Build history of the part. All positions in model axes, mm. A direction names the side the tool comes from. Coordinates: 2 decimals unless noted, no trailing zeros. Write each loop counter-clockwise with the first axis right and the second up, starting at its lowest first coordinate (ties: lowest second). Pieces come first, ordered by that corner, then holes.
```python
from build123d import *

# Parameters (mm, degrees)
F0_W     = 57.99
F0_H     = 6.35
F0_H_2   = 44.45
F1_DEPTH = 6.35
F2_DEPTH = 44.45
F3_R     = 2
F4_DEPTH = 50.801


# Not quite as in the source:
# - a length typed as a fraction of an inch, garbled in the dataset ("3 / 203.2 mm" for 3/8 in), is restored
# - a feature names something its author has since deleted; it is built from what else it names


with BuildPart() as f1:
    # F0 (on Top) → F1 (new body)
    with BuildSketch(Plane.XY):
        with Locations((-9.895, 22.275)):
            Rectangle(F0_W, F0_H)
        with Locations((-9.895, -3.125)):
            Rectangle(F0_W, F0_H_2)
        with BuildLine():
            ThreePointArc((-17.1, -15.5), (-15.5, -13.9), (-13.9, -15.5))
            Line((-13.9, -15.5), (-13.9, -21.75))
            ThreePointArc((-13.9, -21.75), (-15.5, -23.35), (-17.1, -21.75))
            Line((-17.1, -21.75), (-17.1, -15.5))
        make_face(mode=Mode.SUBTRACT)
        with BuildLine():
            ThreePointArc((13.9, -15.5), (15.5, -13.9), (17.1, -15.5))
            Line((17.1, -15.5), (17.1, -21.75))
            ThreePointArc((17.1, -21.75), (15.5, -23.35), (13.9, -21.75))
            Line((13.9, -21.75), (13.9, -15.5))
        make_face(mode=Mode.SUBTRACT)
        with BuildLine():
            ThreePointArc((-11.1, 0), (0, 11.1), (11.1, 0))
            Line((11.1, 0), (11.1, -6.25))
            ThreePointArc((11.1, -6.25), (0, -17.35), (-11.1, -6.25))
            Line((-11.1, -6.25), (-11.1, 0))
        make_face(mode=Mode.SUBTRACT)
        with BuildLine():
            ThreePointArc((-17.1, 15.5), (-15.5, 17.1), (-13.9, 15.5))
            Line((-13.9, 15.5), (-13.9, 9.25))
            ThreePointArc((-13.9, 9.25), (-15.5, 7.65), (-17.1, 9.25))
            Line((-17.1, 9.25), (-17.1, 15.5))
        make_face(mode=Mode.SUBTRACT)
        with BuildLine():
            ThreePointArc((13.9, 15.5), (15.5, 17.1), (17.1, 15.5))
            Line((17.1, 15.5), (17.1, 9.25))
            ThreePointArc((17.1, 9.25), (15.5, 7.65), (13.9, 9.25))
            Line((13.9, 9.25), (13.9, 15.5))
        make_face(mode=Mode.SUBTRACT)
    extrude(amount=F1_DEPTH)

    # F0 (on Top) → F2 (join)
    with BuildSketch(Plane.XY):
        with Locations((-9.895, 22.275)):
            Rectangle(F0_W, F0_H)
    extrude(amount=-F2_DEPTH)

    # F3 (on face) → F4 (cut, through all)
    with BuildSketch(Plane(origin=(0, 25.45, 0), x_dir=(-1, 0, 0), z_dir=(0, 1, 0))):
        with Locations((28.89, -6)):
            Circle(F3_R)
        with Locations((28.89, -38.45)):
            Circle(F3_R)
    extrude(amount=-F4_DEPTH, mode=Mode.SUBTRACT)


solid = f1.part
```
1. Saw through at C-C on y = -9. List the corners of the cut face in (x, z), plus the area to 3 significant figures.
Computed values:
outline: (-38.89, 0) - (-10.75, 0) - (-10.75, 6.35) - (-38.89, 6.35) - close; (10.75, 0) - (19.1, 0) - (19.1, 6.35) - (10.75, 6.35) - close
area: 232 mm2
2. Saw through at A-A on x = -15.5. List the corners of the cut face in (y, z), plus the area to 3 significant figures.
Computed values:
outline: (-25.35, 0) - (-23.35, 0) - (-23.35, 6.35) - (-25.35, 6.35) - close; (-13.9, 0) - (7.65, 0) - (7.65, 6.35) - (-13.9, 6.35) - close; (17.1, 0) - (19.1, 0) - (19.1, -44.45) - (25.45, -44.45) - (25.45, 6.35) - (17.1, 6.35) - close
area: 485 mm2
3. Probe line 1 along Z through (x, y) = (-28.89, 22.75); line 2 along Z through (x, y) = (-28, 20); line 3 along Z through (x, y) = (-24, 3.5). List the from-to ranges inside material, lowest first.
Computed values:
line 1: z = -44.45 to -40.45, -36.45 to -8, -4 to 6.35
line 2: z = -44.45 to -40.24, -36.66 to -7.79, -4.21 to 6.35
line 3: z = 0 to 6.35
4. Flat gauge pins, fed straight in: pin 1 (2 mm diameter, centred on x = -26, y = 8.5, fed in from -Z); pin 2 (6 mm diameter, centred on x = 8.5, z = -22.5, fed in from -Y). Where does each tip first touch, or does it go through?
Computed values:
pin 1: stops at z = 0
pin 2: stops at y = 19.1
5. Mould opens along Y. For faces 4 (the face through (-15.5, -13.9, 3.1)), 5 (the face through (-10, 25.45, -19)), 6 (the face through (-10, -25.35, 3)) say: +Y half, -Y half, draft (parallel to the pull), parting line (faces both ways), or undercut.
Computed values:
face 4: undercut
face 5: +Y half
face 6: -Y half
6. Saw through at D-D on z = -6. List the corners of the cut face in (x, y).
Computed values:
outline: (-38.89, 19.1) - (-30.89, 19.1) - (-30.89, 25.45) - (-38.89, 25.45) - close; (-26.89, 19.1) - (19.1, 19.1) - (19.1, 25.45) - (-26.89, 25.45) - close
7. 3-axis set-ups, long thin cutter, end or side, ignore diameter. For faces 1 (the face through (-38.89, 9, 2)), 2 (the face through (-15.5, 17.1, 3.1)), 3 (the face through (-10, 19.1, -22)): which of +Z, -Z, +X, -X, +Y, -Y reach the whole face in a straight line?
Computed values:
face 1: +Z, -Z, -X, +Y, -Y
face 2: +Z, -Z
face 3: -Z, +X, -X, -Y
8. Saw through at B-B on z = 2. List the corners of the cut face in (x, y), plus the area to 3 significant figures.
Computed values:
outline: (-38.89, -25.35) - (19.1, -25.35) - (19.1, 25.45) - (-38.89, 25.45) - close; hole (-17.1, -21.75) arc R1.6 ccw to (-13.9, -21.75) - (-13.9, -15.5) arc R1.6 ccw to (-17.1, -15.5) - close; hole (-17.1, 9.25) arc R1.6 ccw to (-13.9, 9.25) - (-13.9, 15.5) arc R1.6 ccw to (-17.1, 15.5) - close; hole (-11.1, -6.25) arc R11.1 ccw to (11.1, -6.25) - (11.1, 0) arc R11.1 ccw to (-11.1, 0) - close; hole (13.9, -21.75) arc R1.6 ccw to (17.1, -21.75) - (17.1, -15.5) arc R1.6 ccw to (13.9, -15.5) - close; hole (13.9, 9.25) arc R1.6 ccw to (17.1, 9.25) - (17.1, 15.5) arc R1.6 ccw to (13.9, 15.5) - close
area: 2,310 mm2
